Autodesk Inventor part; units mm, degrees
ref_plane "YZ Plane" through (0, 0, 0) normal (1, 0, 0) x (0, 1, 0)
ref_plane "XZ Plane" through (0, 0, 0) normal (0, 1, 0) x (-1, 0, 0)
ref_plane "XY Plane" through (0, 0, 0) normal (0, 0, 1) x (1, 0, 0)
sketch "Sketch4" plane through (0, 0, 0) normal (0, 1, 0) x (-1, 0, 0)
  line L0 (-127, 152.4) -> (127, 152.4)
  line L1 (127, 152.4) -> (127, -152.4)
  line L2 (127, -152.4) -> (-127, -152.4)
  line L3 (-127, -152.4) -> (-127, 152.4)
  line L4 (-127, 152.4) -> (127, -152.4) construction
  line L5 (127, 152.4) -> (-127, -152.4) construction
  point P0 (0, 0)
  dimension "d6" = 304.8
  dimension "d7" = 254
extrude "Plate1" add sketch "Sketch4" against normal blind 9.525
sketch "Sketch6" plane through (0, 0, 0) normal (0, 1, 0) x (1, 0, 0)
  circle A0 centre (0, 0) radius 29.083
  dimension "d19" = 58.166
extrude "Cut1" cut sketch "Sketch6" against normal blind 9.525
sketch "Sketch7" plane through (0, 0, 0) normal (0, 1, 0) x (1, 0, 0)
  line L0 (-41.275, -101.6) -> (41.275, -101.6)
  line L1 (41.275, -101.6) -> (41.275, 101.6)
  line L2 (41.275, 101.6) -> (-41.275, 101.6)
  line L3 (-41.275, 101.6) -> (-41.275, -101.6)
  line L4 (-41.275, -101.6) -> (41.275, 101.6) construction
  line L5 (41.275, -101.6) -> (-41.275, 101.6) construction
  line L6 (127, 152.4) -> (-127, 152.4)
  point P0 (0, 0)
  point P1 (112.6998, 215.9)
  point P2 (-112.6998, 215.9)
  point P3 (-127, 152.4)
  dimension "d22" = 82.55
  dimension "d23" = 50.8
hole "Hole1" at (-41.275, 0, 101.6) at (41.275, 0, 101.6) at (-41.275, 0, -101.6) at (41.275, 0, -101.6) direction (0, -1, 0) diameter 12.7 depth 9.525
sketch "Sketch8" plane through (0, 0, 0) normal (0, 1, 0) x (1, 0, 0)
  line L0 (-95.25, -120.65) -> (95.25, -120.65)
  line L1 (95.25, -120.65) -> (95.25, 120.65)
  line L2 (95.25, 120.65) -> (-95.25, 120.65)
  line L3 (-95.25, 120.65) -> (-95.25, -120.65)
  line L4 (-95.25, -120.65) -> (95.25, 120.65) construction
  line L5 (95.25, -120.65) -> (-95.25, 120.65) construction
  line L6 (127, -152.4) -> (127, 152.4)
  line L7 (127, 152.4) -> (-127, 152.4)
  point P0 (0, 0)
  dimension "d32" = 31.75
  dimension "d33" = 31.75
hole "Hole2" at (95.25, 0, 120.65) at (95.25, 0, -120.65) at (-95.25, 0, -120.65) at (-95.25, 0, 120.65) direction (0, -1, 0) diameter 12.7 depth 9.525
fillet "Corner Round2" radius 25.4 4 edges at (127, -4.7625, 152.4) (127, -4.7625, -152.4) (-127, -4.7625, 152.4) (-127, -4.7625, -152.4)
equation "\"d20\" = Thickness"
equation "\"d29\" = Thickness"
equation "\"d39\" = Thickness"
equation "\"d8\" = Thickness"
equation "\"BendReliefWidth\" = Thickness"
equation "\"BendReliefDepth\" = 0.5 * Thickness"
equation "\"CornerReliefSize\" = 4 * Thickness"
equation "\"MinimumRemnant\" = 2 * Thickness"
equation "\"TransitionRadius\" = BendRadius"
equation "\"JacobiRadiusSize\" = Thickness"
equation "\"GapSize\" = Thickness"
properties part number "Gooseneck Model-2 Sheet-1" material "SS304"
Input: part model. Units: mm. Frame: model coordinates. Round coordinates to 2 decimals unless told otherwise and drop trailing zeros. Loops run counter-clockwise (first coordinate to the right, second up) from the corner with the lowest first, then second, coordinate; pieces in that order, holes last. Notation, with made-up numbers: (27.5, 65) - (50.5, 65) arc R33 cw to (50.5, 99) - close; hole circle Ø10 at (-4.75, -24). An arc over 180 degrees is marked (long way). One line per item, written item: value. Start each with the question number.
(1) Draft query along X for faces 1 (the cylindrical face through (-43.182, -4.829, 107.657)), 2 (the cylindrical face through (119.36, -4.83, -145.16)), 3 (the cylindrical face through (45.14, -4.83, -106.64)), 4 (the cylindrical face through (-119.36, -4.83, 145.16)). Return one class per face: +X half, -X half, draft (parallel to the pull), parting line (faces both ways), or undercut.
(2) Section A-A, the plane x = 95.25. Return loops of the section in (y, z) (3 decimals).
(3) Section D-D, the plane x = 0. Return loops of the section in (y, z) (3 decimals), plus the area to 3 significant figures.
(4) Ray query, line 1 (Z direction, x = 95.25, y = -5.75); line 2 (X direction, y = -2.75, z = -101.6) (3 decimals); line 3 (X direction, y = -5.75, z = 120.65). Return the intervals inside material, ascending. Write a range as [from, to].
(5) Section C-C, the plane z = -120.65. Return loops of the section in (x, y) (3 decimals), plus the area to 3 significant figures.
(6) Section B-B, the plane z = 0. Return loops of the section in (x, y) (3 decimals), plus the area to 3 significant figures.
Results below:
1. face 1: undercut
1. face 2: +X half
1. face 3: undercut
1. face 4: -X half
2. outline: (-9.525, -152.4) - (0, -152.4) - (0, -127) - (-9.525, -127) - close; (-9.525, -114.3) - (0, -114.3) - (0, 114.3) - (-9.525, 114.3) - close; (-9.525, 127) - (0, 127) - (0, 152.4) - (-9.525, 152.4) - close
3. outline: (-9.525, -152.4) - (0, -152.4) - (0, -29.083) - (-9.525, -29.083) - close; (-9.525, 29.083) - (0, 29.083) - (0, 152.4) - (-9.525, 152.4) - close
3. area: 2,350 mm^2
4. line 1: [-152.4, -127], [-114.3, 114.3], [127, 152.4]
4. line 2: [-127, -47.625], [-34.925, 34.925], [47.625, 127]
4. line 3: [-127, -101.6], [-88.9, 88.9], [101.6, 127]
5. outline: (-127, -9.525) - (-101.6, -9.525) - (-101.6, 0) - (-127, 0) - close; (-88.9, -9.525) - (88.9, -9.525) - (88.9, 0) - (-88.9, 0) - close; (101.6, -9.525) - (127, -9.525) - (127, 0) - (101.6, 0) - close
5. area: 2,180 mm^2
6. outline: (-127, -9.525) - (-29.083, -9.525) - (-29.083, 0) - (-127, 0) - close; (29.083, -9.525) - (127, -9.525) - (127, 0) - (29.083, 0) - close
6. area: 1,870 mm^2
